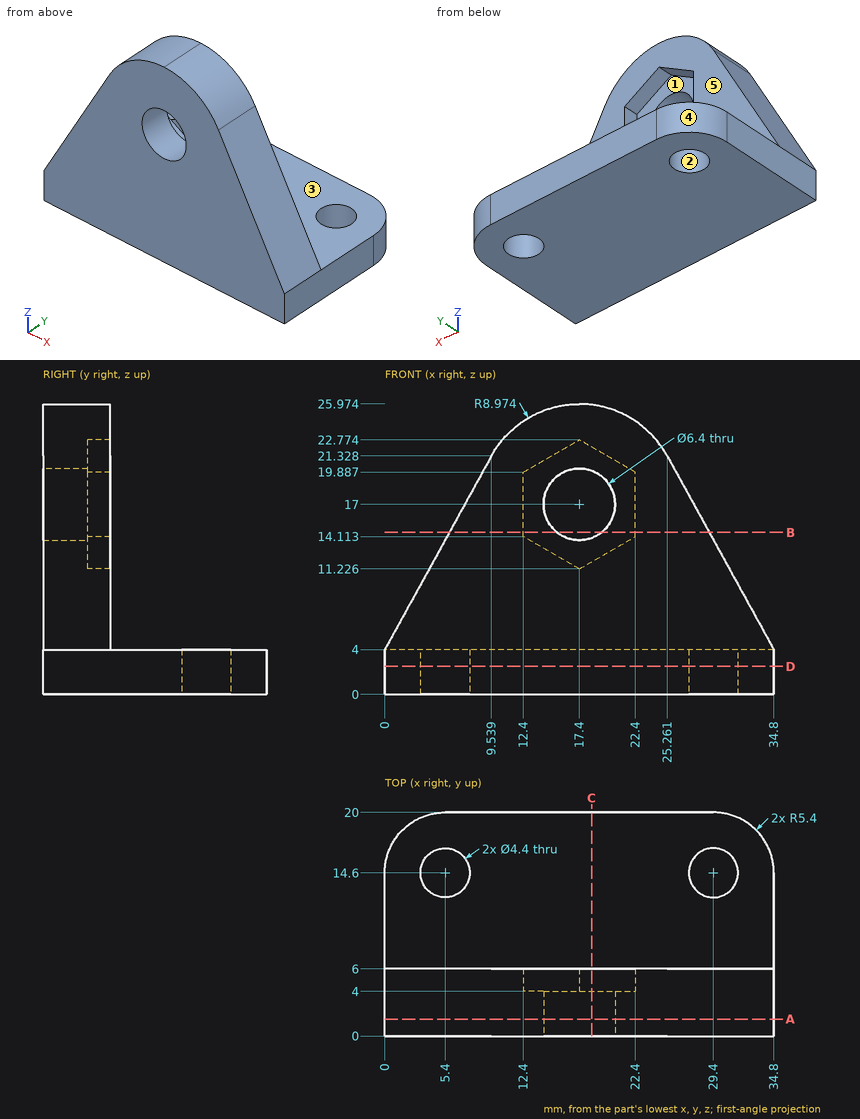
Can you work these out from the drawing? Everything is in mm from the part's minimum corner. A direction names the side the tool comes from. Round coordinates to 2 decimals unless told otherwise and drop trailing zeros. Loops run counter-clockwise (first coordinate to the right, second up) from the corner with the lowest first, then second, coordinate; pieces in that order, holes last. Notation, with made-up numbers: (-32.5, 68.5) - (-11.5, 68.5) arc R20 ccw to (-11.5, 96.5) - close; hole circle Ø2 at (34, 38). An arc over 180 degrees is marked (long way). Answer in a Markdown table with one row per item. Add a question column.
(1) I'm going to push flat-ended pins straight in: pin 1 (6.5 mm diameter, centred on x = 17.5, z = 13, fed in from +Y); pin 2 (4 mm diameter, centred on x = 5.4, y = 14.6, fed in from -Z); pin 3 (1 mm diameter, centred on y = 5.5, z = 18, fed in from +X); pin 4 (2 mm diameter, centred on y = 5, z = 16.5, fed in from -X). Where does each tip first touch, or does it pass through?
(2) If we section it at C-C (x = 18.5): Please give me the cut outline in (y, z) (1 decimal), plus the area to 3 significant figures.
(3) If we mould it in two halves opening along Z, with no side actions, what happens to the marked faces 1, 2 and 3? For each: pulls with the +Z half, pulls with the -Z half, needs draft (parallel to the pull), parting line crosses it, or undercut.
(4) If we section it at B-B (z = 14.5): Please give me the cut outline in (x, y).
(5) If we section it at A-A (y = 1.5): Please give me the cut outline in (x, z), plus the area to 3 significant figures.
(6) If we section it at D-D (z = 2.5): Please give me the cut outline in (x, y), plus the area to 3 significant figures.
(7) For the marked faces 4 and 5, which set-ups out of +Z, -Z, +X, -X, +Y, -Y let a thin tool reach every point of the face, with its end or its side?
(8) I need wall thicknesses on line 1 along Y through (x, z) = (6.5, 13.75); line 2 along X through (y, z) = (2.3, 17) (1 decimal); line 3 along Z through (x, y) = (7, 10.5). Which ranges of each line are inside material? Lowest first, please.
Model answer:
| question | item | result |
|---|---|---|
| 1 | pin 1 | stops at y = 6 |
| 1 | pin 2 | passes through |
| 1 | pin 3 | stops at x = 27.37 |
| 1 | pin 4 | stops at x = 6.33 |
| 2 | outline | (0, 0) - (20, 0) - (20, 4) - (6, 4) - (6, 11.9) - (4, 11.9) - (4, 14) - (0, 14) - close; (0, 20) - (4, 20) - (4, 22.1) - (6, 22.1) - (6, 25.9) - (0, 25.9) - close |
| 2 | area | 167 mm² |
| 3 | face 1 | undercut |
| 3 | face 2 | needs draft |
| 3 | face 3 | pulls with the +Z half |
| 4 | outline | (5.78, 0) - (15.4, 0) - (15.4, 4) - (12.4, 4) - (12.4, 6) - (5.78, 6) - close; (19.4, 0) - (29.02, 0) - (29.02, 6) - (22.4, 6) - (22.4, 4) - (19.4, 4) - close |
| 5 | outline | (0, 0) - (34.8, 0) - (34.8, 4) - (25.26, 21.33) arc R8.97 ccw to (17.4, 25.97) arc R8.97 ccw to (9.54, 21.33) - (0, 4) - close; hole circle Ø6.4 at (17.4, 17) |
| 5 | area | 597 mm² |
| 6 | outline | (0, 0) - (34.8, 0) - (34.8, 14.6) arc R5.4 ccw to (29.4, 20) - (5.4, 20) arc R5.4 ccw to (0, 14.6) - close; hole circle Ø4.4 at (5.4, 14.6); hole circle Ø4.4 at (29.4, 14.6) |
| 6 | area | 653 mm² |
| 7 | face 4 | +Z, -Z, -X, +Y |
| 7 | face 5 | +Z, +X, -X, +Y |
| 8 | line 1 | y = 0 to 6 |
| 8 | line 2 | x = 7.2 to 14.2, 20.6 to 27.6 |
| 8 | line 3 | z = 0 to 4 |
